Study the drawing (mm; zero at the part's minimum x, y, z) and answer. A direction names the side the tool comes from. Give positions to 0.01 mm unless a question says otherwise; leave off trailing zeros. Write each loop counter-clockwise with the first axis right and the second up, starting at its lowest first coordinate (ties: lowest second). Pieces come first, ordered by that corner, then holes. Notation, with made-up numbers: (87, 59.25) -> (136, 59.25) arc R19 ccw to (136, 71.25) -> close; hole circle Ø7 at (42.25, 37.5). An arc over 180 degrees is marked (long way). Put each result on its own line as item: value. Start each with the question number.
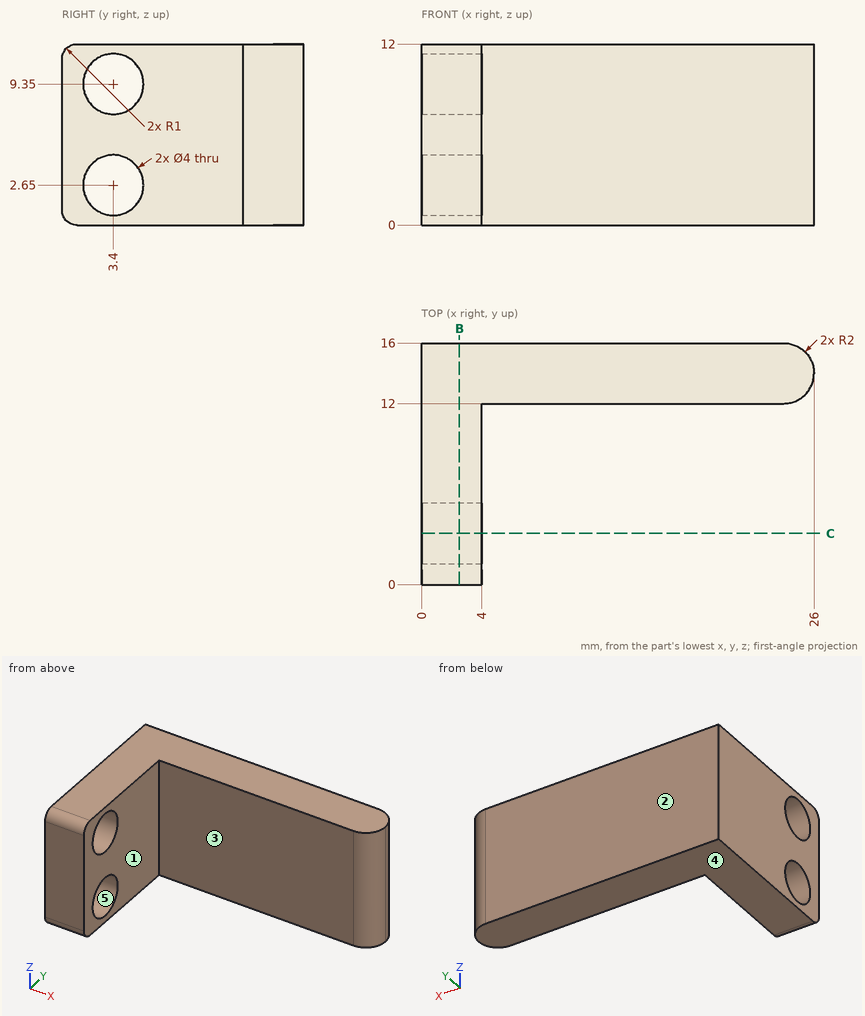
1) Each of these flat-tipped pins is pushed along its axis until it touches: pin 1 Ø3.5 at (y, z) = (5, 8.5) entering from +X; pin 2 Ø3.5 at (x, z) = (15.5, 7.5) entering from -Y; pin 3 Ø5 at (x, y) = (3, 12) entering from -Z. Where does it stop, or does it pass through?
2) Straight lines are drawn through the part: line 1 (Z direction, x = 2.35, y = 3.4); line 2 (Y direction, x = 22.25, z = 2); line 3 (X direction, y = 7.25, z = 3.75). For each, find the intervals that lie inside material, in ascending order. Write a range as [from, to].
3) A cutting plane is placed at C-C on y = 3.4. Give the vertices of the cut face in (x, z), and give its area (3 significant figures).
4) A cutting plane is placed at B-B on x = 2.5. Give the vertices of the cut face in (y, z).
5) For a pull along Z with two mould halves and no side action, classify the marked faces 3, 4 and 5 as pulls with the +Z half, pulls with the -Z half, needs draft (parallel to the pull), parting line crosses it, or undercut.
6) For the marked faces 1 and 2, determine the directions among +Z, -Z, +X, -X, +Y, -Y from which every point of the face is accessible in a straight line to the end or side of a thin tool.
Results found:
1. pin 1: stops at x = 4
1. pin 2: stops at y = 12
1. pin 3: stops at z = 0
2. line 1: z = [0, 0.65], [4.65, 7.35], [11.35, 12]
2. line 2: y = [12, 16]
2. line 3: x = [0, 4]
3. outline: (0, 0) -> (4, 0) -> (4, 0.65) -> (0, 0.65) -> close; (0, 4.65) -> (4, 4.65) -> (4, 7.35) -> (0, 7.35) -> close; (0, 11.35) -> (4, 11.35) -> (4, 12) -> (0, 12) -> close
3. area: 16.0 mm²
4. outline: (0, 1) arc R1 ccw to (1, 0) -> (16, 0) -> (16, 12) -> (1, 12) arc R1 ccw to (0, 11) -> close; hole circle Ø4 at (3.4, 2.65); hole circle Ø4 at (3.4, 9.35)
5. face 3: needs draft
5. face 4: pulls with the -Z half
5. face 5: undercut
6. face 1: +Z, -Z, +X, -Y
6. face 2: +Z, -Z, +X, -X, +Y
